Verification items for the finished model (mm, model axes). Face numbers are marked on the shaded views. Coordinates: 2 decimals unless noted, no trailing zeros. Loops run counter-clockwise (first coordinate to the right, second up) from the corner with the lowest first, then second, coordinate; pieces in that order, holes last. Notation, with made-up numbers: (5, -13.5) - (43, -13.5) arc R18 cw to (43, 8.5) - close; hole circle Ø8 at (82, 30). An arc over 180 degrees is marked (long way). One line per item, written item: value. Start each with the question number.
(1) Section check D-D (y = 17). Record the boundary of the cut face in (x, z).
(2) Section check A-A (y = 9.5). Record the boundary of the cut face in (x, z), plus the area to 3 significant figures.
(3) Section check B-B (z = 11.5). Record the boundary of the cut face in (x, y).
(4) Draft check along X on the marked faces 1, 2, 3 and 4. Enter one of: +X half, -X half, draft (parallel to the pull), parting line (faces both ways), or undercut.
(5) Thickness scan on probe 1 along X at (y, z) = (9, 9.5); probe 2 along Y at (x, z) = (1, 18.5); probe 3 along X at (y, z) = (10, 16.5). Record the ranges inside material, lowest first. Write a range as [from, to].
(6) Gauge pin test, flat ends, axial feed: P1, Ø2, axis at x = 25.5, z = 12, coming from the -Y side; P2, Ø6, axis at x = 33, y = 33, coming from the -Z side. Record the tip position at first contact, or that the pin passes through.
(7) Section check C-C (x = 0). Record the boundary of the cut face in (y, z), plus the area to 3 significant figures.
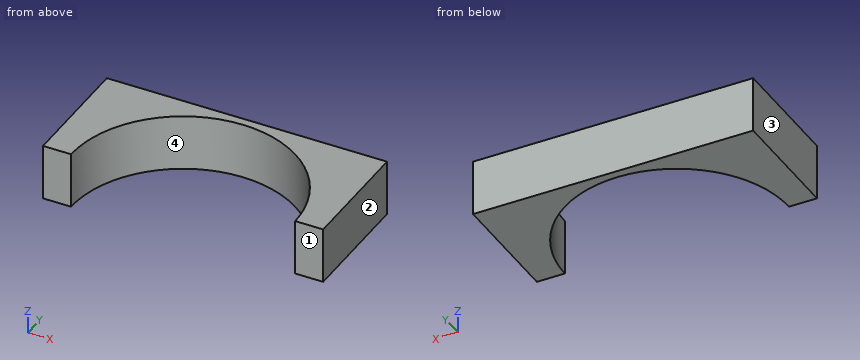
Autodesk Inventor part; units mm, degrees
ref_plane "YZ Plane" through (0, 0, 0) normal (1, 0, 0) x (0, 1, 0)
ref_plane "XZ Plane" through (0, 0, 0) normal (0, 1, 0) x (-1, 0, 0)
ref_plane "XY Plane" through (0, 0, 0) normal (0, 0, 1) x (1, 0, 0)
sketch "Sketch13" plane through (0, 0, 0) normal (0, 0, 1) x (1, 0, 0)
  line L0 (-50, 43) -> (50, 43)
  line L1 (50, 43) -> (50, 0)
  line L2 (50, 0) -> (-50, 0)
  line L3 (-50, 0) -> (-50, 43)
  line L4 (-50, 43) -> (50, 0) construction
  line L5 (50, 43) -> (-50, 0) construction
  point P0 (0, 0)
  point P1 (0, 21.5)
  dimension "d42" = 100
  dimension "d43" = 43
extrude "Extrusion11" add sketch "Sketch13" along normal blind 20
sketch "Sketch14" plane through (0, 0, 20) normal (0, 0, 1) x (1, 0, 0)
  circle A0 centre (0, 0) radius 40
  dimension "d46" = 80
extrude "Extrusion12" cut sketch "Sketch14" against normal blind 50
sketch "Sketch15" plane through (0, 0, 20) normal (0, 0, 1) x (1, 0, 0)
  point P0 (0, 0)
properties part number "pipe_holder_v02"
Responses:
1. outline: (-50, 0) - (-36.21, 0) - (-36.21, 20) - (-50, 20) - close; (36.21, 0) - (50, 0) - (50, 20) - (36.21, 20) - close
2. outline: (-50, 0) - (-38.86, 0) - (-38.86, 20) - (-50, 20) - close; (38.86, 0) - (50, 0) - (50, 20) - (38.86, 20) - close
2. area: 446 mm²
3. outline: (-50, 0) - (-40, 0) arc R40 cw to (40, 0) - (50, 0) - (50, 43) - (-50, 43) - close
4. face 1: draft
4. face 2: +X half
4. face 3: -X half
4. face 4: undercut
5. probe 1: x = [-50, -38.97], [38.97, 50]
5. probe 2: y = [39.99, 43]
5. probe 3: x = [-50, -38.73], [38.73, 50]
6. P1: stops at y = 29.96
6. P2: stops at z = 0
7. outline: (40, 0) - (43, 0) - (43, 20) - (40, 20) - close
7. area: 60.0 mm²
